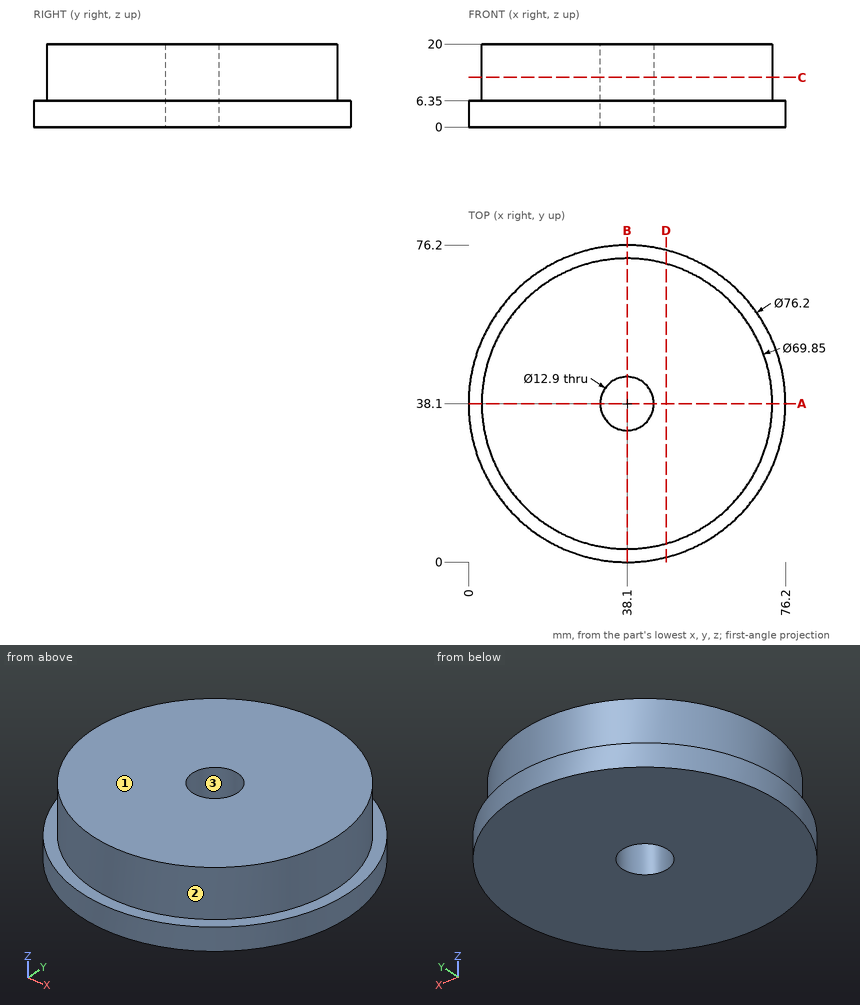
Study the drawing (mm; zero at the part's minimum x, y, z) and answer. Coordinates: 2 decimals unless noted, no trailing zeros. Write each loop counter-clockwise with the first axis right and the second up, starting at its lowest first coordinate (ties: lowest second). Pieces come first, ordered by that corner, then holes. Notation, with made-up numbers: M -29,-37.5 L -23,-37.5 A12 cw -23,-23.5 Z; hole C 25,-23.75 d3. An arc over 180 degrees is marked long. Use a Markdown table: item, result. Add a question column.
1. Section A-A (y = 38.1) is taken. Give the vertices of the cut face in (x, z) (3 decimals), plus the area to 3 significant figures.
2. Given P1, Ø4, axis at x = 31, z = 15, coming from the +Y side; P2, Ø10, axis at x = 42.5, z = 13, coming from the +Y side (3 decimals); P3, Ø12, axis at y = 40.5, z = 17.5, coming from the -X side (3 decimals), each flat-ended and moving along its own axis, determine where each tip first touches the part or whether it passes through.
3. Section C-C (z = 12) is taken. Give the vertices of the cut face in (x, y) (3 decimals).
4. Straight lines are drawn through the part: line 1 along Y through (x, z) = (38, 6.75); line 2 along Y through (x, z) = (38, 3); line 3 along X through (y, z) = (38.1, 12.5) (3 decimals). For each, find the intervals that lie inside material, in ascending order. Write a range as [from, to].
5. For a pull along Y with two mould halves and no side action, classify the marked faces 1, 2 and 3 as +Y half, -Y half, draft (parallel to the pull), parting line (faces both ways), or undercut.
6. Section D-D (x = 47.5) is taken. Give the vertices of the cut face in (y, z), plus the area to 3 significant figures.
Data:
| question | item | result |
|---|---|---|
| 1 | outline | M 0,0 L 31.65,0 L 31.65,20 L 3.175,20 L 3.175,6.35 L 0,6.35 Z; M 44.55,0 L 76.2,0 L 76.2,6.35 L 73.025,6.35 L 73.025,20 L 44.55,20 Z |
| 1 | area | 1,180 mm2 |
| 2 | P1 | stops at y = 72.65 |
| 2 | P2 | stops at y = 73.025 |
| 2 | P3 | stops at x = 3.175 |
| 3 | outline | C 38.1,38.1 d69.85; hole C 38.1,38.1 d12.9 |
| 4 | line 1 | y = [3.18, 31.65], [44.55, 73.02] |
| 4 | line 2 | y = [0, 31.65], [44.55, 76.2] |
| 4 | line 3 | x = [3.175, 31.65], [44.55, 73.025] |
| 5 | face 1 | draft |
| 5 | face 2 | parting line |
| 5 | face 3 | undercut |
| 6 | outline | M 1.18,0 L 75.02,0 L 75.02,6.35 L 71.74,6.35 L 71.74,20 L 4.46,20 L 4.46,6.35 L 1.18,6.35 Z |
| 6 | area | 1,390 mm2 |
